from build123d import *

# Parameters (mm, degrees)
F0_W     = 133.35
F0_H     = 120.65
F1_DEPTH = 19.05
F2_R     = 4.7625
F3_DEPTH = 9.525
F4_R     = 25.4


with BuildPart() as f1:
    # F0 (on Top) → F1 (new body)
    with BuildSketch(Plane.XY):
        Rectangle(F0_W, F0_H)
    extrude(amount=F1_DEPTH)

    # F2 (on face) → F3 (cut)
    with BuildSketch(Plane.XY.offset(19.05)):
        with Locations((-37.11785, 46.229012)):
            Circle(F2_R)
        with Locations((-53.46638, -33.769809)):
            Circle(F2_R)
        with Locations((37.11785, 46.229012)):
            Circle(F2_R)
        with Locations((53.46638, -33.769809)):
            Circle(F2_R)
    extrude(amount=-F3_DEPTH, mode=Mode.SUBTRACT)

    # F4
    f4_edges = [f1.edges().sort_by_distance(p)[0] for p in [
        (66.675, 60.325, 9.525),
        (66.675, -60.325, 9.525),
        (-66.675, -60.325, 9.525),
        (-66.675, 60.325, 9.525),
    ]]
    fillet(f4_edges, radius=F4_R)


solid = f1.part
Read the model definition and answer for the solid it produces. Units are mm, in the model's axes. A direction names the side the tool comes from. Round coordinates to 2 decimals unless told otherwise and drop trailing zeros. Loops run counter-clockwise (first coordinate to the right, second up) from the corner with the lowest first, then second, coordinate; pieces in that order, holes last.
Q1. Section A-A on z = 4.75 is taken. Write down the section's boundary in (x, y) (3 decimals), and give its area (3 significant figures).
Q2. Section B-B on z = 16.75 is taken. Write down the section's boundary in (x, y) (1 decimal), and give its area (3 significant figures).
Q3. Determine the mould class of faces 3 (the face through (-66.675, 0, 9)), 4 (the face through (53, -34, 9.525)), 5 (the face through (-59.43, 52.69, 9.66)) for opening direction Y: released by +Y, released by -Y, zero draft, split by the parting line, or undercut.
Q4. Section D-D on y = -48 is taken. Write down the section's boundary in (x, z), and give its area (3 significant figures).
Q5. Each of these flat-tipped pins is pushed along its axis until it touches: pin 1 (4 mm diameter, centred on x = 50, z = 15.5, fed in from +Y); pin 2 (5 mm diameter, centred on x = 52, y = -33.5, fed in from +Z) (3 decimals). Where does it stop, or does it pass through?
Q6. Consider probe 1 along X at (y, z) = (42.5, 12.5); probe 2 along Y at (x, z) = (40, 13.5) (3 decimals); probe 3 along Y at (x, z) = (-34, 15.75) (3 decimals). Determine where each line is inside the solid, lowest interval first.
Q7. Section C-C on x = -38.5 is taken. Write down the section's boundary in (y, z) (3 decimals).
Q8. Which of the six approach directions +Z, -Z, +X, -X, +Y, -Y give full straight-line access (tool end or side, diameter ignored) to faces 1 (the face through (-57.246, -36.668, 14.354)), 2 (the face through (-59.43, -52.69, 9.66))?
Output:
1. outline: (-66.675, -34.925) arc R25.4 ccw to (-41.275, -60.325) - (41.275, -60.325) arc R25.4 ccw to (66.675, -34.925) - (66.675, 34.925) arc R25.4 ccw to (41.275, 60.325) - (-41.275, 60.325) arc R25.4 ccw to (-66.675, 34.925) - close
1. area: 15,500 mm2
2. outline: (-66.7, -34.9) arc R25.4 ccw to (-41.3, -60.3) - (41.3, -60.3) arc R25.4 ccw to (66.7, -34.9) - (66.7, 34.9) arc R25.4 ccw to (41.3, 60.3) - (-41.3, 60.3) arc R25.4 ccw to (-66.7, 34.9) - close; hole circle Ø9.5 at (-53.5, -33.8); hole circle Ø9.5 at (-37.1, 46.2); hole circle Ø9.5 at (37.1, 46.2); hole circle Ø9.5 at (53.5, -33.8)
2. area: 15,200 mm2
3. face 3: zero draft
3. face 4: undercut
3. face 5: released by +Y
4. outline: (-63.05, 0) - (63.05, 0) - (63.05, 19.05) - (-63.05, 19.05) - close
4. area: 2,400 mm2
5. pin 1: stops at y = 59.42
5. pin 2: stops at z = 9.525
6. probe 1: x = -65.52 to -40.08, -34.16 to 34.16, 40.08 to 65.52
6. probe 2: y = -60.325 to 42.438, 50.02 to 60.325
6. probe 3: y = -60.325 to 42.629, 49.829 to 60.325
7. outline: (-60.325, 0) - (60.325, 0) - (60.325, 19.05) - (50.787, 19.05) - (50.787, 9.525) - (41.671, 9.525) - (41.671, 19.05) - (-60.325, 19.05) - close
8. face 1: +Z
8. face 2: +Z, -Z, -X, -Y
